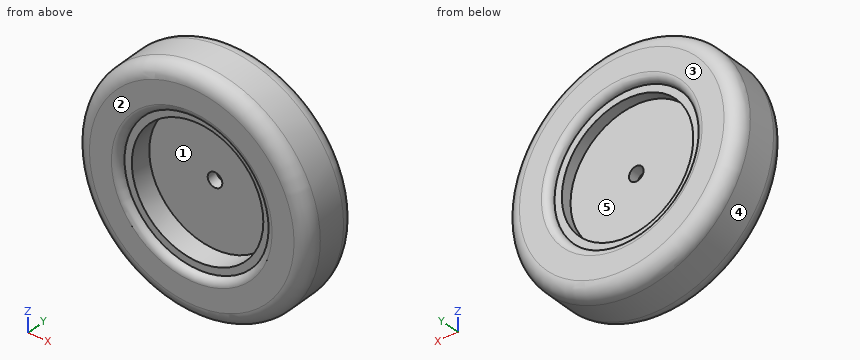
```python
from build123d import *

# Parameters (mm, degrees)
F0_R     = 203.2
F0_R_2   = 127
F1_DEPTH = 50.8
F2_DEPTH = 50.8
F0_R_3   = 114.3
F3_DEPTH = 38.1
F4_DEPTH = 38.1
F5_R     = 25.4
F6_R     = 12.69999
F0_R_4   = 12.7
F7_DEPTH = 19.05


# Not quite as in the source:
# - a fillet or chamfer is up to 0.001 mm smaller than in the source, because OpenCascade refuses the exact size


with BuildPart() as f1:
    # F0 (on Front) → F1 (new body)
    with BuildSketch(Plane.XZ):
        Circle(F0_R)
        Circle(F0_R_2, mode=Mode.SUBTRACT)
    extrude(amount=F1_DEPTH)

    # F0 (on Front) → F2 (join)
    with BuildSketch(Plane.XZ):
        Circle(F0_R)
        Circle(F0_R_2, mode=Mode.SUBTRACT)
    extrude(amount=-F2_DEPTH)

    # F0 (on Front) → F3 (join)
    with BuildSketch(Plane.XZ):
        Circle(F0_R_2)
        Circle(F0_R_3, mode=Mode.SUBTRACT)
    extrude(amount=F3_DEPTH)

    # F0 (on Front) → F4 (join)
    with BuildSketch(Plane.XZ):
        Circle(F0_R_2)
        Circle(F0_R_3, mode=Mode.SUBTRACT)
    extrude(amount=-F4_DEPTH)

    # F5
    f5_edges = [f1.edges().sort_by_distance(p)[0] for p in [
        (-203.2, -50.8, 0),
        (-203.2, 50.8, 0),
    ]]
    fillet(f5_edges, radius=F5_R)

    # F6 (radius 12.7 in the source; OpenCascade refuses exactly that, so slightly less here)
    f6_edges = [f1.edges().sort_by_distance(p)[0] for p in [
        (-127, -50.8, 0),
        (-127, 50.8, 0),
    ]]
    fillet(f6_edges, radius=F6_R)

    # F0 (on Front) → F7 (join)
    with BuildSketch(Plane.XZ):
        Circle(F0_R_3)
        Circle(F0_R_4, mode=Mode.SUBTRACT)
    extrude(amount=-F7_DEPTH)


solid = f1.part
```
Geometry: final body of the model. Coordinates: model frame, mm. Face numbers are marked on the shaded views. A direction names the side the tool comes from. Give positions to 0.01 mm unless a question says otherwise; leave off trailing zeros. Write each loop counter-clockwise with the first axis right and the second up, starting at its lowest first coordinate (ties: lowest second). Pieces come first, ordered by that corner, then holes.
1. Draft query along Z for the marked faces 3, 4 and 5. Return one class per face: released by +Z, released by -Z, zero draft, split by the parting line, or undercut.
2. Line query: probe 1 along Z at (x, y) = (0, 24); probe 2 along X at (y, z) = (37, 101); probe 3 along X at (y, z) = (27.5, 15). Output: solid intervals per line, ascending.
3. Pin query (flat end, axial travel): P1, Ø5, axis at x = 128, z = 150.5, coming from the -Y side; P2, Ø8, axis at x = -52, y = 28, coming from the -Z side; P3, Ø1, axis at y = -23.5, z = 99.5, coming from the +X side. Return the tip coordinate at first contact, or that it passes through.
4. Section query C-C, the plane y = -31.5. Return loops of the section in (x, z).
5. Reachability of the marked faces 1 and 2 from +Z, -Z, +X, -X, +Y, -Y: full face, straight path, thin tool, end or side. Return the list, or none.
Computed:
1. face 3: zero draft
1. face 4: split by the parting line
1. face 5: undercut
2. probe 1: z = -203.2 to -114.3, 114.3 to 203.2
2. probe 2: x = -173.08 to -53.51, 53.51 to 173.08
2. probe 3: x = -202.56 to -113.31, 113.31 to 202.56
3. P1: stops at y = -44.02
3. P2: stops at z = -197.37
3. P3: stops at x = 177.45
4. outline: circle Ø404.91 at (0, 0); hole circle Ø228.6 at (0, 0)
5. face 1: -Y
5. face 2: +Z, -Z, +X, -X, -Y
